Input: part model. Units: mm. Frame: model coordinates. Face numbers are marked on the shaded views. A direction names the side the tool comes from. Give positions to 0.01 mm unless a question says otherwise; leave off trailing zeros. Loops run counter-clockwise (first coordinate to the right, second up) from the corner with the lowest first, then second, coordinate; pieces in that order, holes last. Notation, with made-up numbers: (21, -7) -> (29, -7) arc R9 cw to (29, 9) -> close; hole circle Ø11 at (-23.75, 77). An arc over 180 degrees is marked (long way). Answer as a JSON object with one key per item and string values. Group by question number.
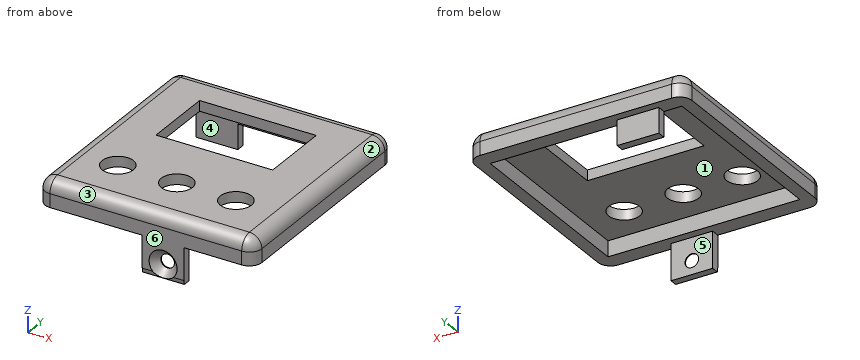
```python
from build123d import *

# Parameters (mm, degrees)
CROQUIS1_W              = 46
CROQUIS1_H              = 46
SALIENTE_EXTRUIR1_DEPTH = 3.75
CROQUIS2_W              = 10
CROQUIS2_H              = 2
SALIENTE_EXTRUIR2_DEPTH = 8.7
CROQUIS5_W              = 10
CROQUIS5_H              = 2
SALIENTE_EXTRUIR3_DEPTH = 6
CROQUIS6_R              = 1.625
CORTAR_EXTRUIR1_DEPTH   = 2
CROQUIS7_R              = 3.35997123
CORTAR_EXTRUIR2_DEPTH   = 1.8
CORTAR_EXTRUIR2_DRAFT   = -44
CORTAR_EXTRUIR3_DEPTH   = 10
CROQUIS10_R             = 3.75
CROQUIS10_W             = 28
CROQUIS10_H             = 17.026229448
SALIENTE_EXTRUIR4_DEPTH = 2.5
REDONDEO1_R             = 3


with BuildPart() as part:
    # Croquis1 → Saliente-Extruir1 (new body)
    with BuildSketch(Plane.XY):
        with BuildLine():
            Line((-25.16229051, 26.433935563), (20.83770949, 26.433935563))
            ThreePointArc((20.83770949, 26.433935563), (22.959029834, 25.555255907), (23.83770949, 23.433935563))
            Line((23.83770949, 23.433935563), (23.83770949, -24.566064437))
            ThreePointArc((23.83770949, -24.566064437), (22.959029834, -26.687384781), (20.83770949, -27.566064437))
            Line((20.83770949, -27.566064437), (-25.16229051, -27.566064437))
            ThreePointArc((-25.16229051, -27.566064437), (-27.283610853, -26.687384781), (-28.16229051, -24.566064437))
            Line((-28.16229051, -24.566064437), (-28.16229051, 23.433935563))
            ThreePointArc((-28.16229051, 23.433935563), (-27.283610853, 25.555255907), (-25.16229051, 26.433935563))
        make_face()
        with Locations((-2.16229051, -0.566064437)):
            Rectangle(CROQUIS1_W, CROQUIS1_H, mode=Mode.SUBTRACT)
    extrude(amount=SALIENTE_EXTRUIR1_DEPTH)

    # Croquis2 → Saliente-Extruir2 (add)
    with BuildSketch(Plane(origin=(0, 0, 0), x_dir=(-1, 0, 0), z_dir=(0, 0, -1))):
        with Locations((-1.97270949, -26.566064437)):
            Rectangle(CROQUIS2_W, CROQUIS2_H)
    extrude(amount=SALIENTE_EXTRUIR2_DEPTH)

    # Croquis5 → Saliente-Extruir3 (add)
    with BuildSketch(Plane(origin=(0, 0, 0), x_dir=(-1, 0, 0), z_dir=(0, 0, -1))):
        with Locations((15.830877534, 23.433935563)):
            Rectangle(CROQUIS5_W, CROQUIS5_H)
    extrude(amount=SALIENTE_EXTRUIR3_DEPTH)

    # Croquis6 → Cortar-Extruir1 (cut)
    with BuildSketch(Plane(origin=(0, -25.566064437, 0), x_dir=(1, 0, 0), z_dir=(0, 1, 0))):
        with Locations(Location((1.97270949, 5.45, 0), (0, 0, 270))):
            Circle(CROQUIS6_R)
    extrude(amount=-CORTAR_EXTRUIR1_DEPTH, mode=Mode.SUBTRACT)


with BuildPart() as cortar_extruir2_tool:
    # Croquis7 → Cortar-Extruir2 (with draft: the straight prism first)
    with BuildSketch(Plane.XZ.offset(27.566064437)):
        with Locations((1.97270949, -5.45)):
            Circle(CROQUIS7_R)
    extrude(amount=-CORTAR_EXTRUIR2_DEPTH)
    # Cortar-Extruir2: the draft: its side faces are tilted about the plane it starts from
    cortar_extruir2_sides = [cortar_extruir2_tool.faces().sort_by_distance(p)[0] for p in [
        (-1.38726174, -26.666064437, -5.45),
    ]]
    draft(cortar_extruir2_sides, Plane.XZ.offset(27.566064437), CORTAR_EXTRUIR2_DRAFT)


with BuildPart() as part_1:
    add(part.part)

    # Cortar-Extruir2: cut by cortar_extruir2_tool
    add(cortar_extruir2_tool.part, mode=Mode.SUBTRACT)

    # Croquis9 → Cortar-Extruir3 (cut)
    with BuildSketch(Plane.ZY.offset(3.02729051)):
        with BuildLine():
            Line((-8.7, -27.375158196), (-8.7, -27.566064437))
            Line((-8.7, -27.566064437), (-7.7, -27.566064437))
            ThreePointArc((-7.7, -27.566064437), (-8.204176074, -27.492486318), (-8.7, -27.375158196))
        make_face()
    extrude(amount=-CORTAR_EXTRUIR3_DEPTH, mode=Mode.SUBTRACT)

    # Croquis10 → Saliente-Extruir4 (add)
    with BuildSketch(Plane.XY.offset(3.75)):
        with BuildLine():
            Line((-25.16229051, 26.433935563), (20.83770949, 26.433935563))
            ThreePointArc((20.83770949, 26.433935563), (22.959029834, 25.555255907), (23.83770949, 23.433935563))
            Line((23.83770949, 23.433935563), (23.83770949, -24.566064437))
            ThreePointArc((23.83770949, -24.566064437), (22.959029834, -26.687384781), (20.83770949, -27.566064437))
            Line((20.83770949, -27.566064437), (-25.16229051, -27.566064437))
            ThreePointArc((-25.16229051, -27.566064437), (-27.283610853, -26.687384781), (-28.16229051, -24.566064437))
            Line((-28.16229051, -24.566064437), (-28.16229051, 23.433935563))
            ThreePointArc((-28.16229051, 23.433935563), (-27.283610853, 25.555255907), (-25.16229051, 26.433935563))
        make_face()
        with Locations((-16.79979051, -14.691064437)):
            Circle(CROQUIS10_R, mode=Mode.SUBTRACT)
        with Locations((-2.63729051, -14.691064437)):
            Circle(CROQUIS10_R, mode=Mode.SUBTRACT)
        with Locations((11.52520949, -14.691064437)):
            Circle(CROQUIS10_R, mode=Mode.SUBTRACT)
        with Locations((-2.773558379, 8.677050287)):
            Rectangle(CROQUIS10_W, CROQUIS10_H, mode=Mode.SUBTRACT)
    extrude(amount=SALIENTE_EXTRUIR4_DEPTH)

    # Redondeo1
    redondeo1_edges = [part_1.edges().sort_by_distance(p)[0] for p in [
        (-27.283610853, 25.555255907, 6.25),
        (-28.16229051, -0.566064437, 6.25),
        (-27.283610853, -26.687384781, 6.25),
        (-2.16229051, -27.566064437, 6.25),
        (22.959029834, -26.687384781, 6.25),
        (23.83770949, -0.566064437, 6.25),
        (22.959029834, 25.555255907, 6.25),
        (-2.16229051, 26.433935563, 6.25),
    ]]
    fillet(redondeo1_edges, radius=REDONDEO1_R)


solid = part_1.part
```
Q1. Section C-C on x = 10. Return the cut outline in (y, z), then the cut area to 3 significant figures.
Q2. Section D-D on y = -8. Return the cut outline in (x, z).
Q3. Set-up query: the marked faces 4, 5 and 6. Return all of +Z, -Z, +X, -X, +Y, -Y with unobstructed straight access to the full face (end or side cutting, diameter ignored); none if empty.
Q4. Section A-A on y = 1. Return the cut outline in (x, z).
Q5. Section B-B on z = 1.75. Return the cut outline in (x, y).
Q6. Pull-direction query (X, two-part tool) for the marked faces 1, 2 and 3; classes: +X half, -X half, draft (parallel to the pull), parting line (faces both ways), or undercut.
Q7. Ray query, probe 1 along Y at (x, z) = (-6.5, 3.5); probe 2 along X at (y, z) = (12, 0.5); probe 3 along X at (y, z) = (-25.7, -5.45). Return the intervals inside material, ascending.
Q8. Pin query (flat end, axial travel): pin 1 Ø0.8 at (y, z) = (11, 4.5) entering from -X; pin 2 Ø4 at (x, z) = (1.97, -5.45) entering from -Y; pin 3 Ø5 at (y, z) = (3, -3) entering from -X; pin 4 Ø2 at (y, z) = (-26.5, -2.5) entering from -X. Return the tip coordinate at first contact, or that it passes through.
Numbers:
{
 "1": {"outline": "(-27.57, 0) -> (-23.57, 0) -> (-23.57, 3.75) -> (-18.12, 3.75) -> (-18.12, 6.25) -> (-24.57, 6.25) arc R3 ccw to (-27.57, 3.25) -> close; (-11.27, 3.75) -> (0.16, 3.75) -> (0.16, 6.25) -> (-11.27, 6.25) -> close; (17.19, 3.75) -> (22.43, 3.75) -> (22.43, 0) -> (26.43, 0) -> (26.43, 3.25) arc R3 ccw to (23.43, 6.25) -> (17.19, 6.25) -> close", "area": "101 mm²"},
 "2": {"outline": "(-28.16, 0) -> (-25.16, 0) -> (-25.16, 3.75) -> (20.84, 3.75) -> (20.84, 0) -> (23.84, 0) -> (23.84, 3.25) arc R3 ccw to (20.84, 6.25) -> (-25.16, 6.25) arc R3 ccw to (-28.16, 3.25) -> close"},
 "3": {"face 4": "-Z", "face 5": "-Z, +X, -X, +Y", "face 6": "+Z, -Z, +X, -X, -Y"},
 "4": {"outline": "(-28.16, 0) -> (-25.16, 0) -> (-25.16, 3.75) -> (-16.77, 3.75) -> (-16.77, 6.25) -> (-25.16, 6.25) arc R3 ccw to (-28.16, 3.25) -> close; (11.23, 3.75) -> (20.84, 3.75) -> (20.84, 0) -> (23.84, 0) -> (23.84, 3.25) arc R3 ccw to (20.84, 6.25) -> (11.23, 6.25) -> close"},
 "5": {"outline": "(-28.16, -24.57) arc R3 ccw to (-25.16, -27.57) -> (20.84, -27.57) arc R3 ccw to (23.84, -24.57) -> (23.84, 23.43) arc R3 ccw to (20.84, 26.43) -> (-25.16, 26.43) arc R3 ccw to (-28.16, 23.43) -> close; hole (-25.16, -23.57) -> (20.84, -23.57) -> (20.84, 22.43) -> (-25.16, 22.43) -> close"},
 "6": {"face 1": "undercut", "face 2": "+X half", "face 3": "draft"},
 "7": {"probe 1": "y = -27.56 to -23.57, 22.43 to 26.42", "probe 2": "x = -28.16 to -25.16, 20.84 to 23.84", "probe 3": "x = -3.03 to 0.35, 3.6 to 6.97"},
 "8": {"pin 1": "stops at x = -28.04", "pin 2": "stops at y = -26.16", "pin 3": "passes through", "pin 4": "stops at x = -3.03"}
}
